from build123d import *

# Parameters (mm, degrees)
SKETCH1_W           = 76.2
SKETCH1_H           = 76.2
SKETCH1_W_2         = 63.5
SKETCH1_H_2         = 63.5
BOSS_EXTRUDE1_DEPTH = 336.55
SKETCH2_R           = 7.9375
CUT_EXTRUDE1_DEPTH  = 77.2


with BuildPart() as part:
    # Sketch1 → Boss-Extrude1 (new body, symmetric)
    with BuildSketch(Plane.XY):
        Rectangle(SKETCH1_W, SKETCH1_H)
        Rectangle(SKETCH1_W_2, SKETCH1_H_2, mode=Mode.SUBTRACT)
    extrude(amount=BOSS_EXTRUDE1_DEPTH, both=True)

    # Sketch2 → Cut-Extrude1 (cut, through all)
    with BuildSketch(Plane(origin=(38.1, 0, 0), x_dir=(0, 0, -1), z_dir=(1, 0, 0))):
        with Locations((298.45, 0)):
            Circle(SKETCH2_R)
    cut_extrude1 = extrude(amount=-CUT_EXTRUDE1_DEPTH, mode=Mode.SUBTRACT)

    # Mirror1: Cut-Extrude1 across plane
    add(cut_extrude1.mirror(Plane.XY), mode=Mode.SUBTRACT)


solid = part.part
CAD build for the part. Positions are in the model's coordinates, mm. A direction names the side the tool comes from. Give positions to 0.01 mm unless a question says otherwise; leave off trailing zeros. Write each loop counter-clockwise with the first axis right and the second up, starting at its lowest first coordinate (ties: lowest second). Pieces come first, ordered by that corner, then holes. Notation, with made-up numbers: (-34.5, 7.25) - (-7.5, 7.25) arc R20 cw to (-7.5, 12.25) - close; hole circle Ø4 at (39.25, 35.5). An arc over 180 degrees is marked (long way). Answer as CSV lines item,"result".
Q1. 3-axis set-ups, long thin cutter, end or side, ignore diameter. For faces 1 (the face through (0, 31.75, 5)), 2 (the face through (35, -3, -305.8)): which of +Z, -Z, +X, -X, +Y, -Y reach the whole face in a straight line?
Result set:
face 1,"+Z, -Z"
face 2,"+X, -X"
Q2. Pull direction X, two halves, no side cores. Call faces 3 (the face through (-34.9, -3, -305.8)), 4 (the face through (-38.1, -1, 5)), 5 (the face through (0, -31.75, 5)): released by +X, released by -X, zero draft, split by the parting line, or undercut.
Result set:
face 3,"zero draft"
face 4,"released by -X"
face 5,"undercut"
Q3. Drill centre lines: line 1 (Y direction, x = -34.5, z = -298.45); line 2 (Y direction, x = 18.5, z = -142.5). Where is each one in solid material? Low to high. Write a range as from..to.
Result set:
line 1,"-38.1..-7.94, 7.94..38.1"
line 2,"-38.1..-31.75, 31.75..38.1"
Q4. Band-saw the part on D-D (z = 141). Give the cut face in (x, y).
Result set:
outline,"(-38.1, -38.1) - (38.1, -38.1) - (38.1, 38.1) - (-38.1, 38.1) - close; hole (-31.75, -31.75) - (31.75, -31.75) - (31.75, 31.75) - (-31.75, 31.75) - close"
Q5. Band-saw the part on C-C (z = 298.45). Give the cut face in (x, y).
Result set:
outline,"(-38.1, -38.1) - (38.1, -38.1) - (38.1, -7.94) - (31.75, -7.94) - (31.75, -31.75) - (-31.75, -31.75) - (-31.75, -7.94) - (-38.1, -7.94) - close; (-38.1, 7.94) - (-31.75, 7.94) - (-31.75, 31.75) - (31.75, 31.75) - (31.75, 7.94) - (38.1, 7.94) - (38.1, 38.1) - (-38.1, 38.1) - close"
Q6. Band-saw the part on A-A (y = 19.5). Give the cut face in (x, z).
Result set:
outline,"(-38.1, -336.55) - (-31.75, -336.55) - (-31.75, 336.55) - (-38.1, 336.55) - close; (31.75, -336.55) - (38.1, -336.55) - (38.1, 336.55) - (31.75, 336.55) - close"
